```python
from build123d import *

# Parameters (mm, degrees)
SKETCH1_W           = 88.9
SKETCH1_H           = 82.55
BOSS_EXTRUDE1_DEPTH = 6.35
SKETCH2_W           = 12.7
SKETCH2_H           = 6.35
SKETCH2_W_2         = 6.35
SKETCH2_H_2         = 25.4
SKETCH2_H_3         = 12.7
CUT_EXTRUDE2_DEPTH  = 6.35


with BuildPart() as part:
    # Sketch1 → Boss-Extrude1 (new body)
    with BuildSketch(Plane.YZ):
        with Locations((44.45, 41.275)):
            Rectangle(SKETCH1_W, SKETCH1_H)
    extrude(amount=BOSS_EXTRUDE1_DEPTH)

    # Sketch2 → Cut-Extrude2 (cut)
    with BuildSketch(Plane.YZ.offset(6.35)):
        with Locations((57.15, 3.175)):
            Rectangle(SKETCH2_W, SKETCH2_H)
        with Locations((31.75, 3.175)):
            Rectangle(SKETCH2_W, SKETCH2_H)
        Polygon((0, 0), (12.7, 0), (12.7, 6.35), (6.35, 6.35), (6.35, 19.05), (0, 19.05), (0, 6.35), align=None)
        Polygon((76.2, 0), (88.9, 0), (88.9, 6.35), (88.9, 19.05), (82.55, 19.05), (82.55, 6.35), (76.2, 6.35), align=None)
        with Locations((3.175, 69.85)):
            Rectangle(SKETCH2_W_2, SKETCH2_H_2)
        with Locations((3.175, 38.1)):
            Rectangle(SKETCH2_W_2, SKETCH2_H_3)
        with Locations((85.725, 38.1)):
            Rectangle(SKETCH2_W_2, SKETCH2_H_3)
        with Locations((85.725, 69.85)):
            Rectangle(SKETCH2_W_2, SKETCH2_H_2)
    extrude(amount=-CUT_EXTRUDE2_DEPTH, mode=Mode.SUBTRACT)


solid = part.part
```
Work out the finished part from the listing and answer in its coordinate system (mm). A direction names the side the tool comes from. Coordinates: 2 decimals unless noted, no trailing zeros. Write each loop counter-clockwise with the first axis right and the second up, starting at its lowest first coordinate (ties: lowest second). Pieces come first, ordered by that corner, then holes. Notation, with made-up numbers: (22, 20.25) - (54, 20.25) arc R24 cw to (54, 53.25) - close; hole circle Ø11 at (51, 36.25). An arc over 180 degrees is marked (long way). Answer as a JSON object with one key per item and string values.
Q1. Consider L1, parallel to Z at x = 4, y = 57. Determine where the line is inside the solid, lowest interval first. Write a range as from..to.
Results list:
{"L1": "z = 6.35..82.55"}
Q2. Which of the six approach directions +Z, -Z, +X, -X, +Y, -Y give full straight-line access (tool end or side, diameter ignored) to faces 4 (the flat face through (3, 10, 6.35)), 5 (the flat face through (3, 86, 57.15)), 6 (the flat face through (3, 76.2, 3))?
Results list:
{"face 4": "-Z, +X, -X, -Y", "face 5": "+Z, +X, -X, +Y", "face 6": "-Z, +X, -X, +Y"}
Q3. Given pin 1 Ø3 at (x, y) = (3, 3) entering from +Z; pin 2 Ø1.9 at (x, z) = (3, 4) entering from -Y; pin 3 Ø3 at (x, y) = (3.5, 57) entering from -Z, each flat-ended and moving along its own axis, determine where each tip first touches the part or whether it passes through.
Results list:
{"pin 1": "stops at z = 57.15", "pin 2": "stops at y = 12.7", "pin 3": "stops at z = 6.35"}
Q4. Find section B-B (z = 76.5). Write down the section's boundary in (x, y).
Results list:
{"outline": "(0, 6.35) - (6.35, 6.35) - (6.35, 82.55) - (0, 82.55) - close"}
Q5. For a pull along Z with two mould halves and no side action, classify faces 1 (the flat face through (3, 82.55, 38)), 2 (the flat face through (3, 44, 0)), 3 (the flat face through (3, 82.55, 13)) as pulls with the +Z half, pulls with the -Z half, needs draft (parallel to the pull), parting line crosses it, or undercut.
Results list:
{"face 1": "undercut", "face 2": "pulls with the -Z half", "face 3": "needs draft"}
